Read the model definition and answer for the solid it produces. Units are mm, in the model's axes. Face numbers are marked on the shaded views. A direction names the side the tool comes from. Round coordinates to 2 decimals unless told otherwise and drop trailing zeros. Write each loop counter-clockwise with the first axis right and the second up, starting at its lowest first coordinate (ties: lowest second). Pieces come first, ordered by that corner, then holes. Notation, with made-up numbers: (66, 80.25) - (88, 80.25) arc R25 cw to (88, 117.25) - close; hole circle Ø6 at (0, 55). An arc over 180 degrees is marked (long way). Answer as CSV lines item,"result". Start each with the question number.
1) Find section C-C on y = 0. Determine the outline of the cut face in (x, z).
2) Find section B-B on z = 3.1. Determine the outline of the cut face in (x, y), then the cut area to 3 significant figures.
3) For a pull along X with two mould halves and no side action, classify the marked faces 1, 2 and 3 as +X half, -X half, draft (parallel to the pull), parting line (faces both ways), or undercut.
4) Find section D-D on x = 20. Determine the outline of the cut face in (y, z), then the cut area to 4 significant figures.
5) This flat-tipped pin is pushed along its axis until it touches: pin 1 (1 mm diameter, centred on y = 2.5, z = 3.5, fed in from +X). Where does it stop, or does it pass through?
6) Consider line 1 along Y through (x, z) = (20, 3.9); line 2 along Y through (x, z) = (5, 3.35); line 3 along X through (y, z) = (-0.75, 5.05). Determine where each line is inside the solid, lowest interval first.
7) Which of the six approach directions +Z, -Z, +X, -X, +Y, -Y give full straight-line access (tool end or side, diameter ignored) to the marked faces 4 and 5?
8) Find section A-A on x = 10.5. Determine the outline of the cut face in (y, z), then the cut area to 3 significant figures.
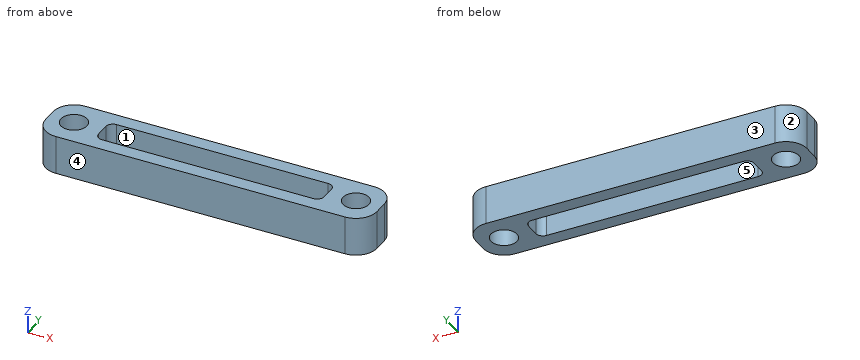
from build123d import *

# Parameters (mm, degrees)
F0_W     = 47
F0_H     = 8
F0_R     = 1.85
F0_W_2   = 32
F0_H_2   = 4
F1_DEPTH = 5.5
F2_R     = 3
F3_R     = 1


with BuildPart() as f1:
    # F0 (on Top) → F1 (new body)
    with BuildSketch(Plane.XY):
        Rectangle(F0_W, F0_H)
        with Locations((-20, 0)):
            Circle(F0_R, mode=Mode.SUBTRACT)
        Rectangle(F0_W_2, F0_H_2, mode=Mode.SUBTRACT)
        with Locations((20, 0)):
            Circle(F0_R, mode=Mode.SUBTRACT)
    extrude(amount=F1_DEPTH)

    # F2
    f2_edges = [f1.edges().sort_by_distance(p)[0] for p in [
        (23.5, -4, 2.75),
        (23.5, 4, 2.75),
        (-23.5, -4, 2.75),
        (-23.5, 4, 2.75),
    ]]
    fillet(f2_edges, radius=F2_R)

    # F3
    f3_edges = [f1.edges().sort_by_distance(p)[0] for p in [
        (-16, 2, 2.75),
        (16, 2, 2.75),
        (16, -2, 2.75),
        (-16, -2, 2.75),
    ]]
    fillet(f3_edges, radius=F3_R)


solid = f1.part
Check values:
1,outline,"(-23.5, 0) - (-21.85, 0) - (-21.85, 5.5) - (-23.5, 5.5) - close; (-18.15, 0) - (-16, 0) - (-16, 5.5) - (-18.15, 5.5) - close; (16, 0) - (18.15, 0) - (18.15, 5.5) - (16, 5.5) - close; (21.85, 0) - (23.5, 0) - (23.5, 5.5) - (21.85, 5.5) - close"
2,outline,"(-23.5, -1) arc R3 ccw to (-20.5, -4) - (20.5, -4) arc R3 ccw to (23.5, -1) - (23.5, 1) arc R3 ccw to (20.5, 4) - (-20.5, 4) arc R3 ccw to (-23.5, 1) - close; hole circle Ø3.7 at (-20, 0); hole (-16, -1) arc R1 ccw to (-15, -2) - (15, -2) arc R1 ccw to (16, -1) - (16, 1) arc R1 ccw to (15, 2) - (-15, 2) arc R1 ccw to (-16, 1) - close; hole circle Ø3.7 at (20, 0)"
2,area,"220 mm^2"
3,face 1,"undercut"
3,face 2,"-X half"
3,face 3,"draft"
4,outline,"(-4, 0) - (-1.85, 0) - (-1.85, 5.5) - (-4, 5.5) - close; (1.85, 0) - (4, 0) - (4, 5.5) - (1.85, 5.5) - close"
4,area,"23.65 mm^2"
5,pin 1,"stops at x = 23.33"
6,line 1,"y = -4 to -1.85, 1.85 to 4"
6,line 2,"y = -4 to -2, 2 to 4"
6,line 3,"x = -23.5 to -21.69, -18.31 to -16, 16 to 18.31, 21.69 to 23.5"
7,face 4,"+Z, -Z, +X, -X, -Y"
7,face 5,"+Z, -Z"
8,outline,"(-4, 0) - (-2, 0) - (-2, 5.5) - (-4, 5.5) - close; (2, 0) - (4, 0) - (4, 5.5) - (2, 5.5) - close"
8,area,"22.0 mm^2"
